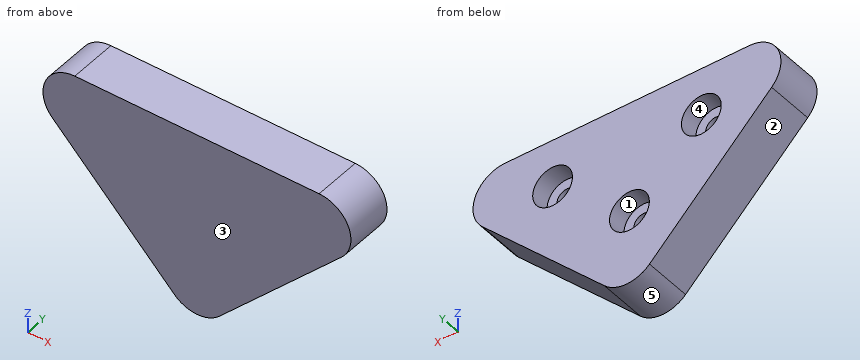
from build123d import *

# Parameters (mm, degrees)
BOSS_EXTRUDE1_DEPTH                            = 3.81
FILLET1_R                                      = 2.54
CBORE_FOR_0_SOCKET_HEAD_CAP_SCREW1_D           = 1.6129
CBORE_FOR_0_SOCKET_HEAD_CAP_SCREW1_DEPTH       = 3.302
CBORE_FOR_0_SOCKET_HEAD_CAP_SCREW1_CBORE_D     = 3.175
CBORE_FOR_0_SOCKET_HEAD_CAP_SCREW1_CBORE_DEPTH = 1.524
CBORE_FOR_0_SOCKET_HEAD_CAP_SCREW1_TIP         = 0.484564046


with BuildPart() as part:
    # Sketch2 → Boss-Extrude1 (new body)
    with BuildSketch(Plane(origin=(0, 0, 0), x_dir=(1, 0, 0), z_dir=(0, 1, 0))):
        Polygon((31.75, 0), (0, 0), (15.875, 15.875), align=None)
    extrude(amount=BOSS_EXTRUDE1_DEPTH)

    # Fillet1
    fillet1_edges = [part.edges().sort_by_distance(p)[0] for p in [
        (0, 1.905, 0),
        (15.875, 1.905, -15.875),
        (31.75, 1.905, 0),
    ]]
    fillet(fillet1_edges, radius=FILLET1_R)

    # CBORE for #0 Socket Head Cap Screw1
    with Locations(Plane(origin=(0, 3.81, 0), x_dir=(1, 0, 0), z_dir=(0, 1, 0))):
        with Locations((9.942102448, 3.81), (15.677428144, 8.89), (21.807897552, 3.81)):
            CounterBoreHole(CBORE_FOR_0_SOCKET_HEAD_CAP_SCREW1_D / 2, CBORE_FOR_0_SOCKET_HEAD_CAP_SCREW1_CBORE_D / 2, CBORE_FOR_0_SOCKET_HEAD_CAP_SCREW1_CBORE_DEPTH, depth=CBORE_FOR_0_SOCKET_HEAD_CAP_SCREW1_DEPTH)
            with Locations((0, 0, -(CBORE_FOR_0_SOCKET_HEAD_CAP_SCREW1_DEPTH + CBORE_FOR_0_SOCKET_HEAD_CAP_SCREW1_TIP / 2))):  # 118° drill point
                Cone(0, CBORE_FOR_0_SOCKET_HEAD_CAP_SCREW1_D / 2, CBORE_FOR_0_SOCKET_HEAD_CAP_SCREW1_TIP, mode=Mode.SUBTRACT)


solid = part.part
Can you work these out from the model? Positions are in its coordinate system, mm. Face numbers are marked on the shaded views. A direction names the side the tool comes from. Round coordinates to 2 decimals unless told otherwise and drop trailing zeros. Write each loop counter-clockwise with the first axis right and the second up, starting at its lowest first coordinate (ties: lowest second). Pieces come first, ordered by that corner, then holes. Notation, with made-up numbers: (2.25, 13) - (40.25, 13) arc R26 cw to (40.25, 42) - close; hole circle Ø6 at (88, -20). An arc over 180 degrees is marked (long way). Write each question's results on one line, items separated by ' | '. Start each with the question number.
1) Which directions (+Z, -Z, +X, -X, +Y, -Y) give clear straight access to the entire face, cutting with the end or side of a thin tool? Please do the marked faces 1 and 2.
2) Please list where these lines run through material, in increasing order: line 1 (X direction, y = 1.4, z = -3.81); line 2 (X direction, y = 2.9, z = -8.89); line 3 (Y direction, x = 17, z = -9.25).
3) For pin 1 Ø3 at (x, z) = (15.68, -8.89) entering from +Y, with a flat end and sliding along its axis, tell me the tip position at first contact or that it passes through.
4) Suppose I cut it at C-C (z = -12.75). List the corners of the cut face in (x, y) for me, and give its area (3 significant figures).
5) Suppose I cut it at A-A (z = -10). List the corners of the cut face in (x, y) for me.
6) Suppose I cut it at B-B (x = 11.25). List the corners of the cut face in (y, z) for me, and give its area (3 significant figures).
7) We'd pull the mould along X, two halves only. Please class the marked faces 3, 4 and 5: released by +X, released by -X, zero draft, split by the parting line, or undercut.
8) Suppose I cut it at D-D (x = 18.25). List the corners of the cut face in (y, z) for me, and give its area (3 significant figures).
Here are the results:
1) face 1: +Y | face 2: -Z, -X, +Y, -Y
2) line 1: x = 3.93 to 9.14, 10.75 to 21, 22.61 to 27.82 | line 2: x = 8.89 to 14.09, 17.26 to 22.86 | line 3: y = 0 to 2.29
3) pin 1: stops at y = 2.29
4) outline: (12.75, 0) - (19, 0) - (19, 3.81) - (12.75, 3.81) - close | area: 23.8 mm2
5) outline: (10, 0) - (21.75, 0) - (21.75, 3.81) - (16.81, 3.81) - (16.81, 2.29) - (14.54, 2.29) - (14.54, 3.81) - (10, 3.81) - close
6) outline: (0, -11.25) - (3.81, -11.25) - (3.81, -4.71) - (2.29, -4.71) - (2.29, -2.91) - (3.81, -2.91) - (3.81, 0) - (0, 0) - close | area: 40.1 mm2
7) face 3: zero draft | face 4: undercut | face 5: split by the parting line
8) outline: (0, -13.5) - (3.81, -13.5) - (3.81, 0) - (0, 0) - close | area: 51.4 mm2
